CAD build for the part. Positions are in the model's coordinates, mm. A direction names the side the tool comes from. Give positions to 0.01 mm unless a question says otherwise; leave off trailing zeros. Loops run counter-clockwise (first coordinate to the right, second up) from the corner with the lowest first, then second, coordinate; pieces in that order, holes last.
Autodesk Inventor part; units mm, degrees
ref_plane "YZ Plane" through (0, 0, 0) normal (1, 0, 0) x (0, 1, 0)
ref_plane "XZ Plane" through (0, 0, 0) normal (0, 1, 0) x (-1, 0, 0)
ref_plane "XY Plane" through (0, 0, 0) normal (0, 0, 1) x (1, 0, 0)
sketch "Skizze1" plane through (0, 0, 0) normal (0, 1, 0) x (-1, 0, 0)
  line L0 (0, 0) -> (0, 32)
  line L1 (0, 32) -> (-23, 32)
  line L2 (-23, 32) -> (-23, 27)
  line L3 (-16, 9) -> (-16, 4)
  line L4 (-16, 4) -> (-20, 4)
  line L5 (-20, 4) -> (-20, 0)
  line L6 (-20, 0) -> (0, 0)
  line L7 (-23, 27) -> (-16, 27)
  line L8 (-16, 27) -> (-16, 25.5)
  line L9 (-16, 25.5) -> (-22.4167, 25.5)
  line L10 (-21.25, 22.5) -> (-16, 22.5)
  line L11 (-16, 22.5) -> (-16, 21)
  line L12 (-16, 21) -> (-20.6667, 21)
  line L13 (-19.5, 18) -> (-16, 18)
  line L14 (-16, 18) -> (-16, 16.5)
  line L15 (-16, 16.5) -> (-18.9167, 16.5)
  line L16 (-17.75, 13.5) -> (-16, 13.5)
  line L17 (-16, 13.5) -> (-16, 12)
  line L18 (-16, 12) -> (-17.1667, 12)
  line L19 (-16, 9) -> (-17.1667, 12)
  line L20 (-17.75, 13.5) -> (-18.9167, 16.5)
  line L21 (-19.5, 18) -> (-20.6667, 21)
  line L22 (-21.25, 22.5) -> (-22.4167, 25.5)
  point P0 (-17.75, 18)
  point P1 (-17.4583, 16.5)
  point P2 (-16.5833, 12)
  point P3 (-16.875, 13.5)
  dimension "d18" = 32
  dimension "d21" = 4
  dimension "d26" = 46
  dimension "d27" = 40
  dimension "d28" = 32
  dimension "d29" = 18
  dimension "d30" = 5
  dimension "d34" = 5
  dimension "d35" = 1.5
  dimension "d36" = 1.5
  dimension "d37" = 1.5
  dimension "d38" = 1.5
  dimension "d42" = 3
  dimension "d43" = 3
  dimension "d44" = 3
revolve "Umdrehung1" add sketch "Skizze1" angle 360 about axis through (0, 0, 0) along (0, 0, 1)
sketch "Skizze2" plane through (0, 0, 32) normal (0, 0, 1) x (1, 0, 0)
  circle A0 centre (0, 0) radius 18 construction
  point P0 (0, -18)
  point P1 (0, 18)
  point P2 (-18, 0)
  point P3 (18, 0)
  dimension "d46" = 36
hole "Bohrung1" at (0, -18, 32) at (0, 18, 32) at (-18, 0, 32) at (18, 0, 32) direction (0, 0, -1) diameter 3.242 depth 9.5
sketch "Skizze3" plane through (0, 0, 32) normal (0, 0, 1) x (1, 0, 0)
  circle A0 centre (0, 0) radius 23
hole "Bohrung2" at (0, 0, 32) direction (0, 0, -1) diameter 27 depth 32
equation "\"d36\" = d35"
equation "\"d37\" = d35"
properties part number "gehaeuse" material "Blei"
1. Probe line 1 along Z through (x, y) = (13, -13.5); line 2 along Z through (x, y) = (-3, 20.5); line 3 along Z through (x, y) = (-18, 5). List the from-to ranges inside material, lowest first.
Responses:
line 1: z = 0 to 4, 16.05 to 16.5, 18 to 21, 22.5 to 25.5, 27 to 32
line 2: z = 22.5 to 25.5, 27 to 32
line 3: z = 0 to 4, 15.9 to 16.5, 18 to 21, 22.5 to 25.5, 27 to 32
2. Pull direction Z, two halves, no side cores. Call faces 5 (the face through (13.1, -4.2, 0)), 6 (the face through (-3.47, 15.62, 21.74)), 7 (the face through (10, -10, 32)), 8 (the face through (-3.484, -15.691, 9.188)): released by +Z, released by -Z, zero draft, split by the parting line, or undercut.
Responses:
face 5: released by -Z
face 6: undercut
face 7: released by +Z
face 8: undercut
3. Drop flat-ended pins along their axis: pin 1 (10 mm diameter, centred on x = 7, y = 16.5, fed in from -Z); pin 2 (6 mm diameter, centred on y = -13, z = 4.5, fed in from +X); pin 3 (1.5 mm diameter, centred on x = 5, z = 11, fed in from -Y); pin 4 (5 mm diameter, centred on y = -17, z = 22, fed in from -X). Give the stop position or say it passes through.
Responses:
pin 1: stops at z = 0
pin 2: stops at x = 17.3
pin 3: stops at y = -16.39
pin 4: stops at x = -15.62
4. Tool access for faces 1 (the face through (13.18, 2.93, 15.78)), 2 (the face through (-0.487, -19.546, 29.465)), 3 (the face through (-5.3, 15.3, 25.5)), 4 (the face through (-4.336, 19.524, 1.972)): list every direction of +Z, -Z, +X, -X, +Y, -Y with a clear straight run to the whole face (end or side of a thin tool).
Responses:
face 1: +Z, -Z
face 2: +Z
face 3: none
face 4: -Z
5. Saw through at A-A, the plane x = 0. Count the separate pieces of the cut face and the enclosed holes in it, and give its area (3 significant figures).
Responses:
separate pieces: 6
enclosed holes: 0
area: 287 mm2
6. Saw through at D-D, the plane z = 10.5. List the corners of the cut face in (x, y).
Responses:
outline: circle Ø33.17 at (0, 0); hole circle Ø27 at (0, 0)
7. Saw through at C-C, the plane z = 6. List the corners of the cut face in (x, y), and give its area (3 significant figures).
Responses:
outline: circle Ø32 at (0, 0); hole circle Ø27 at (0, 0)
area: 232 mm2
